```python
from build123d import *

# Parameters (mm, degrees)
SCHIZZO1_W                   = 29
SCHIZZO1_H                   = 35
ESTRUSIONE_ESTRUSIONE1_DEPTH = 5
SCHIZZO2_W                   = 29
SCHIZZO2_H                   = 5
ESTRUSIONE_ESTRUSIONE2_DEPTH = 80
SCHIZZO4_W                   = 16
SCHIZZO4_H                   = 6
TAGLIO_ESTRUSIONE2_DEPTH     = 10


with BuildPart() as part:
    # Schizzo1 → Estrusione-Estrusione1 (new body)
    with BuildSketch(Plane.XY):
        Rectangle(SCHIZZO1_W, SCHIZZO1_H)
    extrude(amount=ESTRUSIONE_ESTRUSIONE1_DEPTH)

    # Schizzo2 → Estrusione-Estrusione2 (add)
    with BuildSketch(Plane.XY.offset(5)):
        with Locations((0, -15)):
            Rectangle(SCHIZZO2_W, SCHIZZO2_H)
    extrude(amount=ESTRUSIONE_ESTRUSIONE2_DEPTH)

    # Schizzo4 → Taglio-Estrusione2 (cut)
    with BuildSketch(Plane(origin=(0, -12.5, 0), x_dir=(1, 0, 0), z_dir=(0, 1, 0))):
        with Locations((0, -39.5)):
            Rectangle(SCHIZZO4_W, SCHIZZO4_H)
        with Locations((0, -74.5)):
            Rectangle(SCHIZZO4_W, SCHIZZO4_H)
    extrude(amount=-TAGLIO_ESTRUSIONE2_DEPTH, mode=Mode.SUBTRACT)


solid = part.part
```
The listing builds one solid part. Answer for the finished solid, in the listing's coordinates (mm). A direction names the side the tool comes from. Give positions to 0.01 mm unless a question says otherwise; leave off trailing zeros. Write each loop counter-clockwise with the first axis right and the second up, starting at its lowest first coordinate (ties: lowest second). Pieces come first, ordered by that corner, then holes. Notation, with made-up numbers: (-7.5, 7) -> (26.5, 7) arc R24 cw to (26.5, 40) -> close; hole circle Ø10 at (-24.75, 47.5). An arc over 180 degrees is marked (long way). Use one line per item in the form item = value.
1) Section B-B on x = 5.75 is taken. Write down the section's boundary in (y, z), plus the area to 3 significant figures.
Result:
outline = (-17.5, 0) -> (17.5, 0) -> (17.5, 5) -> (-12.5, 5) -> (-12.5, 36.5) -> (-17.5, 36.5) -> close; (-17.5, 42.5) -> (-12.5, 42.5) -> (-12.5, 71.5) -> (-17.5, 71.5) -> close; (-17.5, 77.5) -> (-12.5, 77.5) -> (-12.5, 85) -> (-17.5, 85) -> close
area = 515 mm²
2) A tool of negligible diameter and unlimited length cuts with its end or side. For faces 1 (the flat face through (14.5, -13, 33)), 2 (the flat face through (0, -12.5, 44)), 3 (the flat face through (0, -15, 77.5)), from which of +Z, -Z, +X, -X, +Y, -Y can it reach the whole face along a straight path? Write none if from no direction.
Result:
face_1 = +Z, -Z, +X, +Y, -Y
face_2 = +Z, +X, -X, +Y
face_3 = +Y, -Y
3) Section D-D on z = 52 is taken. Write down the section's boundary in (x, y), plus the area to 3 significant figures.
Result:
outline = (-14.5, -17.5) -> (14.5, -17.5) -> (14.5, -12.5) -> (-14.5, -12.5) -> close
area = 145 mm²
4) For a pull along Z with two mould halves and no side action, classify faces 4 (the flat face through (0, 3, 5)), 5 (the flat face through (-8, -15, 75)), 6 (the flat face through (0, 0, 0)) as +Z half, -Z half, draft (parallel to the pull), parting line (faces both ways), or undercut.
Result:
face_4 = +Z half
face_5 = undercut
face_6 = -Z half
5) Each of these flat-tipped pins is pushed along its axis until it touches: P1, Ø3, axis at x = 10.5, y = 7, coming from the -Z side; P2, Ø8.5, axis at x = -6, z = 52, coming from the +Y side; P3, Ø1, axis at x = 4.5, y = 1.5, coming from the +Z side. Where does it stop, or does it pass through?
Result:
P1 = 0
P2 = -12.5
P3 = 5
6) Section A-A on z = 37.5 is taken. Write down the section's boundary in (x, y).
Result:
outline = (-14.5, -17.5) -> (-8, -17.5) -> (-8, -12.5) -> (-14.5, -12.5) -> close; (8, -17.5) -> (14.5, -17.5) -> (14.5, -12.5) -> (8, -12.5) -> close
7) Section C-C on x = -11 is taken. Write down the section's boundary in (y, z).
Result:
outline = (-17.5, 0) -> (17.5, 0) -> (17.5, 5) -> (-12.5, 5) -> (-12.5, 85) -> (-17.5, 85) -> close
8) Straight lines are drawn through the part: probe 1 along Z at (x, y) = (-7, -13.5); probe 2 along Y at (x, z) = (10, 75.5); probe 3 along Z at (x, y) = (-1.75, 15). For each, find the intervals that lie inside material, in ascending order.
Result:
probe_1 = 0 to 36.5, 42.5 to 71.5, 77.5 to 85
probe_2 = -17.5 to -12.5
probe_3 = 0 to 5
